from build123d import *

# Parameters (mm, degrees)
SKETCH1_W                = 101.6
SKETCH1_H                = 152.4
BOSS_EXTRUDE1_DEPTH      = 6.35
SKETCH2_W                = 38.1
SKETCH2_H                = 63.5
CUT_EXTRUDE1_DEPTH       = 92.800885072
BOSS_EXTRUDE3_DEPTH      = 10.0965
BOSS_EXTRUDE3_DEPTH_BACK = 6.35
CUT_EXTRUDE2_REACH       = 105.862
SKETCH6_R                = 3
SKETCH7_W                = 24.005
SKETCH7_H                = 2.009
BOSS_EXTRUDE4_DEPTH      = 16.4465
BOSS_EXTRUDE5_REACH      = 129.401
SKETCH10_W               = 13
SKETCH10_H               = 6.35
CUT_EXTRUDE3_REACH       = 138.165
SKETCH11_W               = 13
SKETCH11_H               = 10.0965
BOSS_EXTRUDE6_DEPTH      = 10
CUT_EXTRUDE4_DEPTH       = 2.54
SKETCH14_W               = 101.6
SKETCH14_H               = 6.35
BOSS_EXTRUDE7_DEPTH      = 50.8
SKETCH15_W               = 19.05
SKETCH15_H               = 19.05
BOSS_EXTRUDE8_DEPTH      = 66.04
SKETCH16_W               = 19.05
SKETCH16_H               = 19.05
BOSS_EXTRUDE9_DEPTH      = 6.35
SKETCH17_W               = 184.15
SKETCH17_H               = 72.39
BOSS_EXTRUDE10_DEPTH     = 6.35


with BuildPart() as part:
    # Sketch1 → Boss-Extrude1 (new body)
    with BuildSketch(Plane(origin=(0, 0, 0), x_dir=(1, 0, 0), z_dir=(0, 1, 0))):
        Rectangle(SKETCH1_W, SKETCH1_H)
    extrude(amount=-BOSS_EXTRUDE1_DEPTH)

    # Sketch2 → Cut-Extrude1 (cut, through all)
    with BuildSketch(Plane(origin=(0, 0, 0), x_dir=(1, 0, 0), z_dir=(0, 1, 0))):
        Rectangle(SKETCH2_W, SKETCH2_H)
    extrude(amount=-CUT_EXTRUDE1_DEPTH, mode=Mode.SUBTRACT)

    # Sketch4 → Boss-Extrude3 (add, two sides: drawn at the far end of the back side and taken through both)
    with BuildSketch(Plane(origin=(0, 0, 0), x_dir=(1, 0, 0), z_dir=(0, 1, 0)).offset(-BOSS_EXTRUDE3_DEPTH_BACK)):
        Polygon((61.595, -8.509), (50.8, -8.509), (50.8, -14.859), (67.945, -14.859), (67.945, 14.859), (50.8, 14.859), (50.8, 8.509), (61.595, 8.509), align=None)
        Polygon((50.8, -8.509), (21.59, -8.509), (21.59, 8.509), (50.8, 8.509), (50.8, 14.859), (19.05, 14.859), (19.05, -14.859), (50.8, -14.859), align=None)
    extrude(amount=BOSS_EXTRUDE3_DEPTH + BOSS_EXTRUDE3_DEPTH_BACK)

    # Sketch6 → Cut-Extrude2 (cut, up to next)
    with BuildSketch(Plane.ZY.offset(-19.05), mode=Mode.PRIVATE) as cut_extrude2_sk1:
        with Locations((0, 10.0965)):
            Circle(SKETCH6_R)
    cut_extrude2_tool1 = extrude(cut_extrude2_sk1.sketch, amount=-CUT_EXTRUDE2_REACH, mode=Mode.PRIVATE) & part.part
    add(cut_extrude2_tool1.solids().sort_by_distance((19.05, 10.0965, 0))[0], mode=Mode.SUBTRACT)

    # Sketch7 → Boss-Extrude4 (add, through all)
    with BuildSketch(Plane(origin=(0, 10.0965, 0), x_dir=(1, 0, 0), z_dir=(0, 1, 0))):
        with Locations((49.5925, 7.5045)):
            Rectangle(SKETCH7_W, SKETCH7_H)
        with Locations((49.5925, -7.5045)):
            Rectangle(SKETCH7_W, SKETCH7_H)
    extrude(amount=-BOSS_EXTRUDE4_DEPTH)

    # Sketch10 → Boss-Extrude5 (add, up to next)
    with BuildSketch(Plane(origin=(50.8, 0, 0), x_dir=(0, 0, -1), z_dir=(1, 0, 0)), mode=Mode.PRIVATE) as boss_extrude5_sk1:
        with Locations((0, -3.175)):
            Rectangle(SKETCH10_W, SKETCH10_H)
    boss_extrude5_tool1 = extrude(boss_extrude5_sk1.sketch, amount=BOSS_EXTRUDE5_REACH, mode=Mode.PRIVATE) - part.part
    add(boss_extrude5_tool1.solids().sort_by_distance((50.8, -3.175, 0))[0])

    # Sketch11 → Cut-Extrude3 (cut, up to next)
    with BuildSketch(Plane.ZY.offset(-61.595), mode=Mode.PRIVATE) as cut_extrude3_sk1:
        with Locations((0, 5.04825)):
            Rectangle(SKETCH11_W, SKETCH11_H)
    cut_extrude3_tool1 = extrude(cut_extrude3_sk1.sketch, amount=-CUT_EXTRUDE3_REACH, mode=Mode.PRIVATE) & part.part
    add(cut_extrude3_tool1.solids().sort_by_distance((61.595, 5.04825, 0))[0], mode=Mode.SUBTRACT)

    # Sketch12 → Boss-Extrude6 (add)
    with BuildSketch(Plane(origin=(0, 10.0965, 0), x_dir=(1, 0, 0), z_dir=(0, 1, 0))):
        Polygon((67.945, -14.859), (67.945, -6.5), (37.59, -6.5), (37.59, -8.509), (21.59, -8.509), (21.59, -3), (19.05, -3), (19.05, -14.859), align=None)
        Polygon((37.59, 6.5), (67.945, 6.5), (67.945, 14.859), (19.05, 14.859), (19.05, 3), (21.59, 3), (21.59, 8.509), (37.59, 8.509), align=None)
    extrude(amount=BOSS_EXTRUDE6_DEPTH)

    # Sketch13 → Cut-Extrude4 (cut)
    with BuildSketch(Plane.ZY.offset(-19.05)):
        Polygon((3, 10.0965), (7, 10.0965), (7, 14.0965), (11, 14.0965), (11, 17.0965), (7, 17.0965), (7, 20.0965), (3, 20.0965), align=None)
    cut_extrude4 = extrude(amount=-CUT_EXTRUDE4_DEPTH, mode=Mode.SUBTRACT)

    # Mirror1: Cut-Extrude4 across plane
    add(cut_extrude4.mirror(Plane.XY), mode=Mode.SUBTRACT)

    # Sketch14 → Boss-Extrude7 (add)
    with BuildSketch(Plane(origin=(0, 0, -76.2), x_dir=(-1, 0, 0), z_dir=(0, 0, -1))):
        with Locations((0, -3.175)):
            Rectangle(SKETCH14_W, SKETCH14_H)
    extrude(amount=BOSS_EXTRUDE7_DEPTH)

    # Sketch15 → Boss-Extrude8 (add)
    with BuildSketch(Plane.XZ.offset(6.35)):
        with Locations((-60.325, 66.675)):
            Rectangle(SKETCH15_W, SKETCH15_H)
        with Locations((60.325, 66.675)):
            Rectangle(SKETCH15_W, SKETCH15_H)
        with Locations((-41.275, -117.475)):
            Rectangle(SKETCH15_W, SKETCH15_H)
        with Locations((41.275, -117.475)):
            Rectangle(SKETCH15_W, SKETCH15_H)
    extrude(amount=BOSS_EXTRUDE8_DEPTH)


with BuildPart() as boss_extrude8_piece_1:
    # of the separate pieces the step leaves, piece 1, a body of its own (boss_extrude8_pieces)
    add(part.part.solids().sort_by_distance((-50.8, 0, 76.2))[0])



with BuildPart() as boss_extrude8_piece_2:
    # of the separate pieces the step leaves, piece 2, a body of its own (boss_extrude8_pieces)
    add(part.part.solids().sort_by_distance((-50.8, -72.39, 76.2))[0])


with BuildPart() as boss_extrude8_piece_3:
    # of the separate pieces the step leaves, piece 3, a body of its own (boss_extrude8_pieces)
    add(part.part.solids().sort_by_distance((50.8, -72.39, 76.2))[0])


with BuildPart() as boss_extrude8_piece_1_1:
    add(boss_extrude8_piece_1.part)

    add(boss_extrude8_piece_2.part)  # Boss-Extrude9 merges Boss-Extrude8 piece 2

    add(boss_extrude8_piece_3.part)  # Boss-Extrude9 merges Boss-Extrude8 piece 3
    # Sketch16 → Boss-Extrude9 (add)
    with BuildSketch(Plane(origin=(0, -6.35, 0), x_dir=(1, 0, 0), z_dir=(0, 1, 0))):
        with Locations((60.325, -66.675)):
            Rectangle(SKETCH16_W, SKETCH16_H)
        with Locations((-60.325, -66.675)):
            Rectangle(SKETCH16_W, SKETCH16_H)
    extrude(amount=BOSS_EXTRUDE9_DEPTH)

    # Sketch17 → Boss-Extrude10 (add)
    with BuildSketch(Plane.ZY.offset(50.8)):
        with Locations((-34.925, -36.195)):
            Rectangle(SKETCH17_W, SKETCH17_H)
    extrude(amount=BOSS_EXTRUDE10_DEPTH)


solid = boss_extrude8_piece_1_1.part
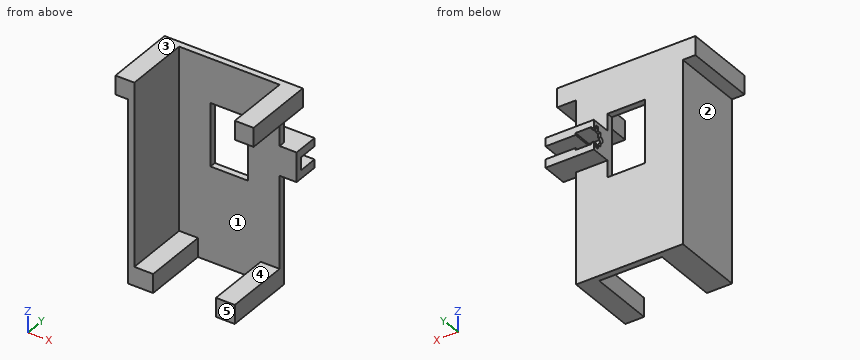
Part model, mm, in its own coordinate system. Face numbers are marked on the shaded views. A direction names the side the tool comes from. Round coordinates to 2 decimals unless told otherwise and drop trailing zeros. Loops run counter-clockwise (first coordinate to the right, second up) from the corner with the lowest first, then second, coordinate; pieces in that order, holes last. Notation, with made-up numbers: (73.25, -7.5) - (101.25, -7.5) arc R35 cw to (101.25, 25.5) - close; hole circle Ø5 at (51.25, 68.25). An arc over 180 degrees is marked (long way). Answer as a JSON object with one key per item and string values.
Item 1: Pin check, flat tips, straight feed: pin 1 (10 mm diameter, centred on x = -45.5, y = -14.5, fed in from +Z); pin 2 (20 mm diameter, centred on y = -53.5, z = -19, fed in from +X); pin 3 (9.5 mm diameter, centred on y = -50.5, z = -118, fed in from -X). Stop position of each tip, or through.
Output:
{"pin 1": "z = -107.95", "pin 2": "x = -50.8", "pin 3": "x = -57.15"}
Item 2: Pull direction X, two halves, no side cores. Call the marked faces 1, 2 and 3: pulls with the +X half, pulls with the -X half, needs draft (parallel to the pull), parting line crosses it, or undercut.
Output:
{"face 1": "undercut", "face 2": "pulls with the -X half", "face 3": "needs draft"}
Item 3: Band-saw the part on D-D on z = -65.5. List the corners of the cut face in (x, y), plus the area to 3 significant figures.
Output:
{"outline": "(-57.15, -72.39) - (-50.8, -72.39) - (-50.8, -6.35) - (50.8, -6.35) - (50.8, 0) - (-57.15, 0) - close", "area": "1,100 mm2"}
Item 4: Wall check: L1, parallel to Z at x = 58, y = 0.5; L2, parallel to X at y = -14, z = 68.5; L3, parallel to X at y = -49.5, z = -109. Give the ranges that are in metal, low to high.
Output:
{"L1": "-14.86 to -6.5, 6.5 to 14.86", "L2": "-69.85 to -50.8, 50.8 to 69.85", "L3": "-57.15 to -31.75, 31.75 to 50.8"}
Item 5: Band-saw the part on A-A on x = -4.5. List the corners of the cut face in (y, z).
Output:
{"outline": "(-6.35, -127) - (0, -127) - (0, -31.75) - (-6.35, -31.75) - close; (-6.35, 31.75) - (0, 31.75) - (0, 76.2) - (-6.35, 76.2) - close"}
Item 6: Band-saw the part on B-B on y = -44. List the corners of the cut face in (x, z), plus the area to 3 significant figures.
Output:
{"outline": "(-69.85, 57.15) - (-57.15, 57.15) - (-57.15, -127) - (-31.75, -127) - (-31.75, -107.95) - (-50.8, -107.95) - (-50.8, 76.2) - (-69.85, 76.2) - close; (31.75, -127) - (50.8, -127) - (50.8, -107.95) - (31.75, -107.95) - close; (50.8, 57.15) - (69.85, 57.15) - (69.85, 76.2) - (50.8, 76.2) - close", "area": "2,620 mm2"}
Item 7: Tool access for the marked faces 4 and 5: list every direction of +Z, -Z, +X, -X, +Y, -Y with a clear straight run to the whole face (end or side of a thin tool).
Output:
{"face 4": "+Z, +X, -Y", "face 5": "+Z, -Z, +X, -X, -Y"}
